from build123d import *

# Parameters (mm, degrees)
SKETCH1_W                = 30
SKETCH1_H                = 10
MAIN_DEPTH               = 25
SKETCH5_R                = 1.05
SKETCH5_R_2              = 7.15
MAINANDFIXHOLE_DEPTH     = 11
SKETCH6_R                = 2.2
CODERFIXHOLE2_DEPTH      = 1.5
CODERHOLE2_DEPTH         = 7
SKETCH10_W               = 32
SKETCH10_H               = 16
LINK_DEPTH               = 4
SKETCH8_R                = 1.25
VERTICALHOLES_DEPTH      = 10
HOLELPATTERN1_COUNT      = 2
HOLELPATTERN1_PITCH      = 25
HOLELPATTERN1_COUNT_DIR2 = 2
HOLELPATTERN1_PITCH_DIR2 = 10
SKETCH13_R               = 2.5
LINKREINFORCEMENT_DEPTH  = 2
FILLET6_R                = 12
SKETCH14_R               = 1.25
FIXHOLE_DEPTH            = 10
SKETCH16_R               = 1.75
HEXAKEYACCESSHOLE_DEPTH  = 15


with BuildPart() as part:
    # Sketch1 → Main (new body)
    with BuildSketch(Plane.XY):
        Rectangle(SKETCH1_W, SKETCH1_H)
    extrude(amount=MAIN_DEPTH)

    # Sketch5 → MainAndFixHole (cut, through all)
    with BuildSketch(Plane(origin=(0, -5, 0), x_dir=(-1, 0, 0), z_dir=(0, -1, 0))):
        with Locations((0, -21.5)):
            Circle(SKETCH5_R)
        with Locations((-8.227241336, -7.25)):
            Circle(SKETCH5_R)
        with Locations((8.227241336, -7.25)):
            Circle(SKETCH5_R)
        with Locations((0, -12)):
            Circle(SKETCH5_R_2)
    extrude(amount=-MAINANDFIXHOLE_DEPTH, mode=Mode.SUBTRACT)

    # Sketch6 → CoderFixHole2 (cut)
    with BuildSketch(Plane(origin=(0, 5, 0), x_dir=(-1, 0, 0), z_dir=(0, -1, 0))):
        with Locations((0, -21.5)):
            Circle(SKETCH6_R)
        with Locations((-8.227241336, -7.25)):
            Circle(SKETCH6_R)
        with Locations((8.227241336, -7.25)):
            Circle(SKETCH6_R)
    extrude(amount=CODERFIXHOLE2_DEPTH, mode=Mode.SUBTRACT)

    # Sketch11 → CoderHole2 (cut)
    with BuildSketch(Plane(origin=(0, -5, 0), x_dir=(1, 0, 0), z_dir=(0, 1, 0))):
        with BuildLine():
            Line((-15, 0), (15, 0))
            Line((15, 0), (15, -17))
            Line((15, -17), (10.908712115, -17))
            ThreePointArc((10.908712115, -17), (0, -24), (-10.908712115, -17))
            Line((-10.908712115, -17), (-15, -17))
            Line((-15, -17), (-15, 0))
        make_face()
    extrude(amount=CODERHOLE2_DEPTH, mode=Mode.SUBTRACT)

    # Sketch10 → Link (add)
    with BuildSketch(Plane.XY.offset(25)):
        with Locations((0, -1)):
            Rectangle(SKETCH10_W, SKETCH10_H)
    extrude(amount=LINK_DEPTH)

    # Sketch8 → VerticalHoles (cut)
    with BuildSketch(Plane.XY.offset(29)):
        with Locations((12.5, 4)):
            Circle(SKETCH8_R)
    verticalholes = extrude(amount=-VERTICALHOLES_DEPTH, mode=Mode.SUBTRACT)

    # HoleLPattern1: VerticalHoles 2 × 2
    with Locations(*[(-i * HOLELPATTERN1_PITCH, -j * HOLELPATTERN1_PITCH_DIR2, 0) for i in range(HOLELPATTERN1_COUNT) for j in range(HOLELPATTERN1_COUNT_DIR2) if (i, j) != (0, 0)]):
        add(verticalholes, mode=Mode.SUBTRACT)

    # Sketch13 → LinkReinforcement (add)
    with BuildSketch(Plane(origin=(0, 0, 25), x_dir=(-1, 0, 0), z_dir=(0, 0, -1))):
        with Locations((-12.5, -6)):
            Circle(SKETCH13_R)
        with Locations((12.5, -6)):
            Circle(SKETCH13_R)
    extrude(amount=LINKREINFORCEMENT_DEPTH)

    # Fillet6
    fillet6_edges = [part.edges().sort_by_distance(p)[0] for p in [
        (-15, 3.5, 0),
        (15, 3.5, 0),
    ]]
    fillet(fillet6_edges, radius=FILLET6_R)

    # Sketch14 → FixHole (cut)
    with BuildSketch(Plane.XY.offset(29)):
        with Locations((-12.5, -6)):
            Circle(SKETCH14_R)
        with Locations((12.5, -6)):
            Circle(SKETCH14_R)
    extrude(amount=-FIXHOLE_DEPTH, mode=Mode.SUBTRACT)

    # Sketch16 → HexaKeyAccessHole (cut)
    with BuildSketch(Plane.XY.offset(29)):
        with Locations((-5.5, 3.5)):
            Circle(SKETCH16_R)
        with Locations((5.5, 3.5)):
            Circle(SKETCH16_R)
    extrude(amount=-HEXAKEYACCESSHOLE_DEPTH, mode=Mode.SUBTRACT)


solid = part.part
Could you check a few things on this model? Use its own coordinates, in mm. A direction names the side the tool comes from. Give positions to 0.01 mm unless a question says otherwise; leave off trailing zeros. Order: outer loops, then holes, each group sorted by start corner. A loop starts at its lowest first (then second) coordinate and runs counter-clockwise, first axis right, second up. Notation, with made-up numbers: M 18.5,72.25 L 22.5,72.25 A16 ccw 22.5,77.25 Z; hole C 0,37 d3. An arc over 180 degrees is marked long. One line per question, with ' | ' between items.
1. I want a section at C-C (y = -0.5). List the corners of the cut face in (x, z) for me, and give its area (3 significant figures).
Results:
outline: M -16,25 L -15,25 L -15,17 L -10.91,17 A12 cw 10.91,17 L 15,17 L 15,25 L 16,25 L 16,29 L -16,29 Z | area: 258 mm²
2. We'd pull the mould along X, two halves only. Please class faces 1 (the face through (11.39, 3.52, 3.42)), 2 (the face through (-4, -5, 24)), 3 (the face through (13, -2, 17)): +X half, -X half, draft (parallel to the pull), parting line (faces both ways), or undercut.
Results:
face 1: +X half | face 2: undercut | face 3: draft
3. I want a section at A-A (z = 26). List the corners of the cut face in (x, y) for me, and give its area (3 significant figures).
Results:
outline: M -16,-9 L 16,-9 L 16,7 L -16,7 Z; hole C -12.5,-6 d2.5; hole C -12.5,4 d2.5; hole C -5.5,3.5 d3.5; hole C 5.5,3.5 d3.5; hole C 12.5,-6 d2.5; hole C 12.5,4 d2.5 | area: 473 mm²
4. I want a section at B-B (x = -12.5). List the corners of the cut face in (y, z) for me, and give its area (3 significant figures).
Results:
outline: M -9,25 L -8.5,25 L -8.5,23 L -7.25,23 L -7.25,29 L -9,29 Z; M -5,17 L 2,17 L 2,4.67 L 5,4.67 L 5,19 L 2.75,19 L 2.75,29 L -4.75,29 L -4.75,19 L -5,19 Z; M 5.25,25 L 7,25 L 7,29 L 5.25,29 Z | area: 148 mm²
5. For faces 4 (the face through (0, -2, 24)), 5 (the face through (12.23, 2.78, 24.07)), 6 (the face through (-15, 1, 20)), 7 (the face through (-6.61, 4.26, 5.76)), which set-ups out of +Z, -Z, +X, -X, +Y, -Y let a thin tool reach every point of the face, with its end or its side?
Results:
face 4: -Z, -Y | face 5: +Z | face 6: -Z, -X, +Y, -Y | face 7: +Y
6. I want a section at D-D (z = 7.25). List the corners of the cut face in (x, y) for me.
Results:
outline: M -14.02,2 L -9.28,2 L -9.28,3.5 L -10.43,3.5 L -10.43,5 L -14.02,5 Z; M -7.18,2 L -5.34,2 L -5.34,5 L -6.03,5 L -6.03,3.5 L -7.18,3.5 Z; M 5.34,2 L 7.18,2 L 7.18,3.5 L 6.03,3.5 L 6.03,5 L 5.34,5 Z; M 9.28,2 L 14.02,2 L 14.02,5 L 10.43,5 L 10.43,3.5 L 9.28,3.5 Z
7. I'm going to push flat-ended pins straight in: pin 1 (1.3 mm diameter, centred on x = 0, z = 21.5, fed in from +Y); pin 2 (10 mm diameter, centred on x = -3, z = 9, fed in from -Y); pin 3 (1.2 mm diameter, centred on x = 12.5, y = -2.5, fed in from -Z); pin 4 (2 mm diameter, centred on x = 7.5, y = 2, fed in from -Z). Where does each tip first touch, or does it pass through?
Results:
pin 1: through | pin 2: y = 2 | pin 3: z = 17 | pin 4: z = 0.52
8. If I drill on line 1 (Y direction, x = 12.5, z = 26); line 2 (Y direction, x = 11.5, z = 27.5); line 3 (Z direction, x = 0, y = 3.15), over which ranges is the centre line in solid material (lowest first)?
Results:
line 1: -9 to -7.25, -4.75 to 2.75, 5.25 to 7 | line 2: -9 to -6.75, -5.25 to 3.25, 4.75 to 7 | line 3: 0 to 4.85, 19.15 to 20.45, 22.55 to 29
